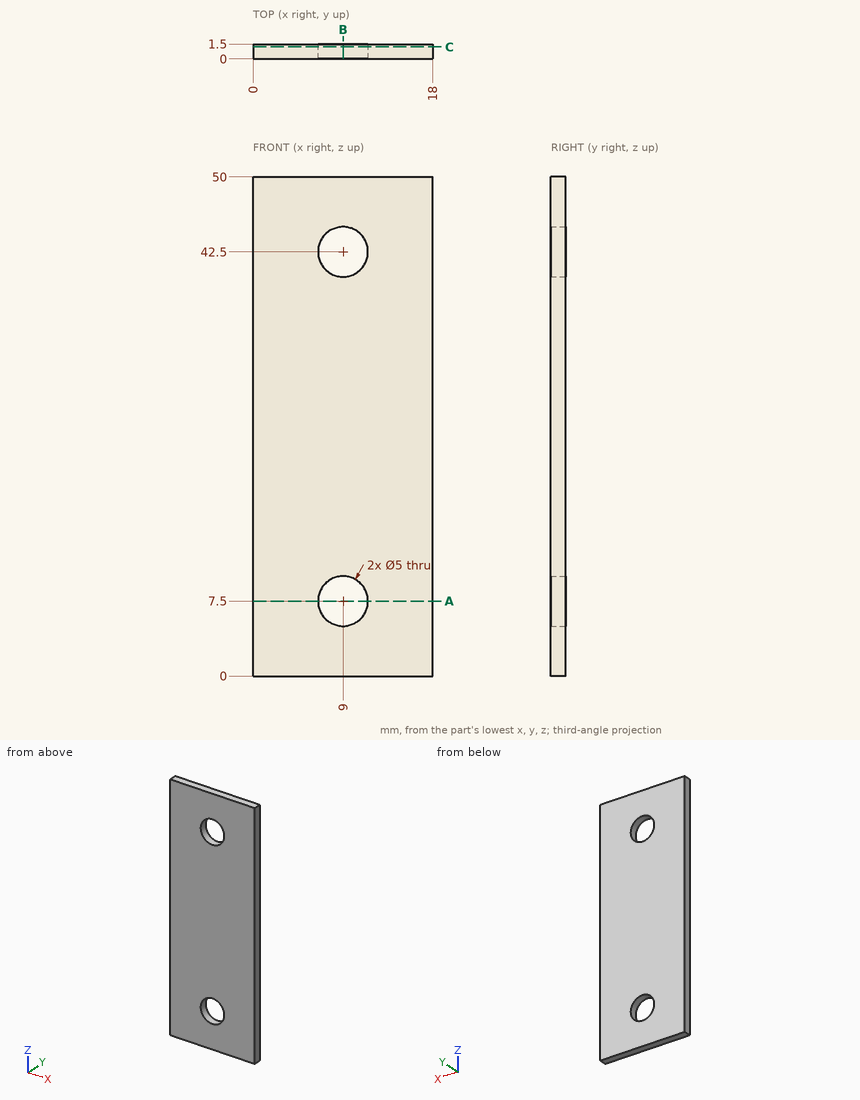
Input: dimensioned drawing with shaded views. Units: mm. Origin: part minimum x, y, z. Give positions to 0.01 mm unless a question says otherwise; leave off trailing zeros. Write each loop counter-clockwise with the first axis right and the second up, starting at its lowest first coordinate (ties: lowest second). Pieces come first, ordered by that corner, then holes. Notation, with made-up numbers: (9.25, -33) - (38.25, -33) arc R15 ccw to (38.25, -12) - close; hole circle Ø4 at (60.25, 25). An arc over 180 degrees is marked (long way). One line per item, written item: value. Start each with the question number.
Q1. Section query B-B, the plane x = 9. Return the cut outline in (y, z).
Q2. Section query A-A, the plane z = 7.5. Return the cut outline in (x, y), then the cut area to 3 significant figures.
Q3. Material intervals for probe 1 along Z at (x, y) = (9, 0.45); probe 2 along Z at (x, y) = (8.25, 0.65); probe 3 along X at (y, z) = (1.35, 6.5), sorted ascending. Write a range as from..to.
Q4. Section query C-C, the plane y = 1.2. Return the cut outline in (x, z), then the cut area to 3 significant figures.
Answer:
1. outline: (0, 0) - (1.5, 0) - (1.5, 5) - (0, 5) - close; (0, 10) - (1.5, 10) - (1.5, 40) - (0, 40) - close; (0, 45) - (1.5, 45) - (1.5, 50) - (0, 50) - close
2. outline: (0, 0) - (6.5, 0) - (6.5, 1.5) - (0, 1.5) - close; (11.5, 0) - (18, 0) - (18, 1.5) - (11.5, 1.5) - close
2. area: 19.5 mm2
3. probe 1: z = 0..5, 10..40, 45..50
3. probe 2: z = 0..5.12, 9.88..40.12, 44.88..50
3. probe 3: x = 0..6.71, 11.29..18
4. outline: (0, 0) - (18, 0) - (18, 50) - (0, 50) - close; hole circle Ø5 at (9, 7.5); hole circle Ø5 at (9, 42.5)
4. area: 861 mm2
